Here's how the part is built. I have some questions about the finished solid (model axes, mm). Round coordinates to 2 decimals unless told otherwise and drop trailing zeros. Loops run counter-clockwise (first coordinate to the right, second up) from the corner with the lowest first, then second, coordinate; pieces in that order, holes last. Notation, with made-up numbers: M -17.75,66 L 38.25,66 A31 cw 38.25,95 Z; hole C 87,5.25 d11. An arc over 180 degrees is marked long. Put each result on its own line as item: value. Start each with the question number.
```python
from build123d import *

# Parameters (mm, degrees)
BOSS_EXTRUDE1_DEPTH = 214.686455
CUT_EXTRUDE3_DEPTH  = 32.423010849
SKETCH5_W           = 20
SKETCH5_H           = 5
SKETCH5_W_2         = 3
SKETCH5_H_2         = 20
BOSS_EXTRUDE2_DEPTH = 5


with BuildPart() as part:
    # Sketch2 → Boss-Extrude1 (new body)
    with BuildSketch(Plane.XY.offset(4.949356739)):
        Polygon((-52.961538618, -36.862052104), (-51.252736373, -41.56098761), (-128.567156233, -69.67694155), (-130.275958479, -64.978006044), align=None)
    extrude(amount=BOSS_EXTRUDE1_DEPTH)

    # Sketch4 → Cut-Extrude3 (cut, through all)
    with BuildSketch(Plane(origin=(7.362313595, -20.245196221, 0), x_dir=(-0.939787101, -0.341760449, 0), z_dir=(0.341760449, -0.939787101, 0))):
        Polygon((101.40457011, -4.949356739), (105.60457011, -4.949356739), (105.60457011, -8.949356739), (107.30457011, -8.949356739), (107.30457011, -11.749356739), (105.60457011, -11.749356739), (105.60457011, -21.749356739), (101.40457011, -21.749356739), (101.40457011, -11.749356739), (99.70457011, -11.749356739), (99.70457011, -8.949356739), (101.40457011, -8.949356739), align=None)
        Polygon((62.37056233, -60.720970532), (62.37056233, -56.520970532), (66.37056233, -56.520970532), (66.37056233, -54.820970532), (69.17056233, -54.820970532), (69.17056233, -56.520970532), (79.17056233, -56.520970532), (79.17056233, -60.720970532), (69.17056233, -60.720970532), (69.17056233, -62.420970532), (66.37056233, -62.420970532), (66.37056233, -60.720970532), align=None)
        Polygon((105.60457011, -219.635811913), (101.40457011, -219.635811913), (101.40457011, -215.635811913), (99.70457011, -215.635811913), (99.70457011, -212.835811913), (101.40457011, -212.835811913), (101.40457011, -202.835811913), (105.60457011, -202.835811913), (105.60457011, -212.835811913), (107.30457011, -212.835811913), (107.30457011, -215.635811913), (105.60457011, -215.635811913), align=None)
        Polygon((66.37056233, -168.064198119), (66.37056233, -169.764198119), (69.17056233, -169.764198119), (69.17056233, -168.064198119), (79.17056233, -168.064198119), (79.17056233, -163.864198119), (69.17056233, -163.864198119), (69.17056233, -162.164198119), (66.37056233, -162.164198119), (66.37056233, -163.864198119), (62.37056233, -163.864198119), (62.37056233, -168.064198119), align=None)
        Polygon((144.638577891, -163.864198119), (144.638577891, -168.064198119), (140.638577891, -168.064198119), (140.638577891, -169.764198119), (137.838577891, -169.764198119), (137.838577891, -168.064198119), (127.838577891, -168.064198119), (127.838577891, -163.864198119), (137.838577891, -163.864198119), (137.838577891, -162.164198119), (140.638577891, -162.164198119), (140.638577891, -163.864198119), align=None)
        Polygon((140.638577891, -56.520970532), (140.638577891, -54.820970532), (137.838577891, -54.820970532), (137.838577891, -56.520970532), (127.838577891, -56.520970532), (127.838577891, -60.720970532), (137.838577891, -60.720970532), (137.838577891, -62.420970532), (140.638577891, -62.420970532), (140.638577891, -60.720970532), (144.638577891, -60.720970532), (144.638577891, -56.520970532), align=None)
    extrude(amount=-CUT_EXTRUDE3_DEPTH, mode=Mode.SUBTRACT)

    # Sketch5 → Boss-Extrude2 (add)
    with BuildSketch(Plane(origin=(7.362313595, -20.245196221, 0), x_dir=(0.939787101, 0.341760449, 0), z_dir=(0.341760449, -0.939787101, 0))):
        with Locations((-81.88756622, 2.449356739)):
            Rectangle(SKETCH5_W, SKETCH5_H)
        with Locations((-125.121574, 2.449356739)):
            Rectangle(SKETCH5_W, SKETCH5_H)
        with Locations((-60.87056233, 112.292584326)):
            Rectangle(SKETCH5_W_2, SKETCH5_H_2)
        with Locations((-60.87056233, 193.850005016)):
            Rectangle(SKETCH5_W_2, SKETCH5_H_2)
        with Locations((-81.88756622, 222.135811913)):
            Rectangle(SKETCH5_W, SKETCH5_H)
        with Locations((-125.121574, 222.135811913)):
            Rectangle(SKETCH5_W, SKETCH5_H)
    extrude(amount=-BOSS_EXTRUDE2_DEPTH)


solid = part.part
```
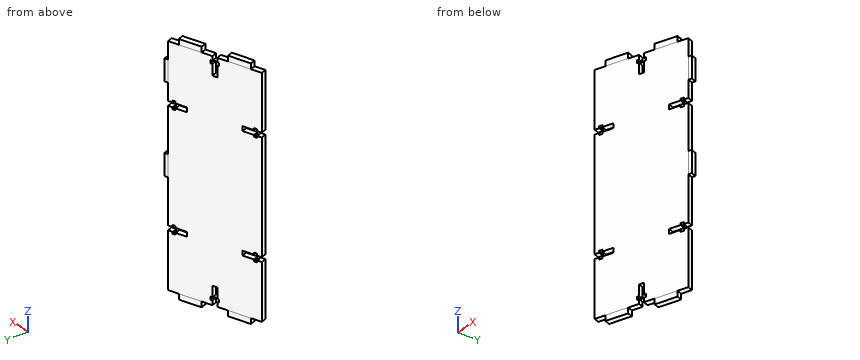
1) Suppose I cut it at A-A (z = 19). Write out the boundary of the cut face in (x, y).
2) Suppose I cut it at C-C (z = 89.5). Write out the boundary of the cut face in (x, y), plus the area to 3 significant figures.
3) Suppose I cut it at B-B (x = -105.5). Write out the boundary of the cut face in (y, z), plus the area to 3 significant figures.
4) If I drill on probe 1 along Y at (x, z) = (-102, 63.5); probe 2 along X at (y, z) = (-68, 56); probe 3 along Y at (x, z) = (-100, 89), over which ranges is the centre line in solid material (lowest first)? Write a range as from..to.
5) I'm going to push flat-ended pins straight in: P1, Ø3.5, axis at x = -125, y = -66.5, coming from the -Z side; P2, Ø2, axis at x = -56.5, y = -41, coming from the +Z side; P3, Ø10, axis at y = -60.5, z = 110, coming from the -X side. Where does each tip first touch, or does it pass through?
Results are:
1. outline: M -130.28,-64.98 L -128.57,-69.68 L -91.88,-56.34 L -93.59,-51.64 Z; M -89.65,-50.2 L -87.94,-54.9 L -51.25,-41.56 L -52.96,-36.86 Z
2. outline: M -130.28,-64.98 L -128.57,-69.68 L -51.25,-41.56 L -52.96,-36.86 Z
2. area: 411 mm²
3. outline: M -61.29,-0.05 L -55.97,-0.05 L -55.97,224.64 L -61.29,224.64 Z
3. area: 1,200 mm²
4. probe 1: -60.02..-54.7
4. probe 2: -129.18..-124.92
4. probe 3: -59.29..-53.97
5. P1: z = 4.95
5. P2: z = 219.64
5. P3: x = -130.28
